```python
from build123d import *

# Parameters (mm, degrees)
FILLET1_R  = 0.4
SLOTSKE_W  = 3
SLOTSKE_H  = 0.6
SLOT_DEPTH = 0.5


with BuildPart() as part:
    # BodySke → BaseBody (revolve)
    with BuildSketch(Plane.XY):
        Polygon((0, 0), (0, 1.5), (0.324017858, 1.5), (1, 0.8), (8, 0.8), (8, 0), align=None)
    revolve(axis=Axis((0, 0, 0), (1, 0, 0)))

    # Fillet1
    fillet1_edges = [part.edges().sort_by_distance(p)[0] for p in [
        (1, -0.8, 0),
    ]]
    fillet(fillet1_edges, radius=FILLET1_R)

    # SlotSke → Slot (cut)
    with BuildSketch(Plane.ZY):
        Rectangle(SLOTSKE_W, SLOTSKE_H)
    extrude(amount=-SLOT_DEPTH, mode=Mode.SUBTRACT)


solid = part.part
```
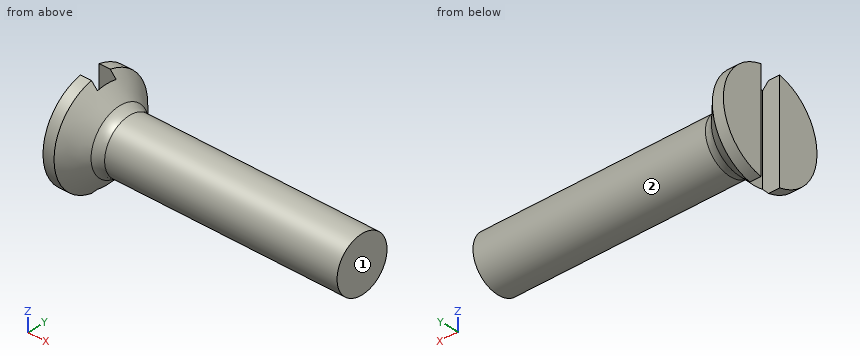
Source: CAD feature listing. Evaluate the final solid. Frame: model axes, mm. Face numbers are marked on the shaded views. A direction names the side the tool comes from. Coordinates: 2 decimals unless noted, no trailing zeros. Order: outer loops, then holes, each group sorted by start corner. A loop starts at its lowest first (then second) coordinate and runs counter-clockwise, first axis right, second up. Notation, with made-up numbers: (-21, -36) - (9, -36) arc R16 cw to (9, -21) - close; hole circle Ø1 at (5, 5.5). An arc over 180 degrees is marked (long way). One line per item, written item: value.
1) Cut plane A-A on x = 3.75. Output: boundary loops of the cut face in (y, z).
Computed values:
outline: circle Ø1.6 at (0, 0)
2) Contact query for flat-ended pins moving along their axis: pin 1 (1 mm diameter, centred on y = 0.5, z = -0.5, fed in from -X); pin 2 (1.5 mm diameter, centred on x = 3, y = -0.5, fed in from +Z); pin 3 (0.5 mm diameter, centred on y = 0, z = 0, fed in from -X); pin 4 (1 mm diameter, centred on x = 2, z = -1, fed in from +Y). Output: stop coordinate, or through.
Computed values:
pin 1: stops at x = 0
pin 2: stops at z = 0.8
pin 3: stops at x = 0.5
pin 4: stops at y = 0.62
3) Reachability of the marked faces 1 and 2 from +Z, -Z, +X, -X, +Y, -Y: full face, straight path, thin tool, end or side. Return the list, or none.
Computed values:
face 1: +Z, -Z, +X, +Y, -Y
face 2: +X
4) Ray query, line 1 (Y direction, x = 6.5, z = 0); line 2 (X direction, y = -0.1, z = 0.2); line 3 (X direction, y = -1.2, z = -0.55). Return the intervals inside material, ascending. Write a range as [from, to].
Computed values:
line 1: y = [-0.8, 0.8]
line 2: x = [0.5, 8]
line 3: x = [0, 0.5]
